Could you check a few things on this model? Use its own coordinates, in mm. Face numbers are marked on the shaded views. A direction names the side the tool comes from. Give positions to 0.01 mm unless a question says otherwise; leave off trailing zeros. Write each loop counter-clockwise with the first axis right and the second up, starting at its lowest first coordinate (ties: lowest second). Pieces come first, ordered by that corner, then holes. Notation, with made-up numbers: (-17, 29) -> (18, 29) arc R18 ccw to (18, 43) -> close; hole circle Ø10 at (62.25, 74.5). An arc over 180 degrees is marked (long way). Write item = value, one per line. Start each with the question number.
```python
from build123d import *

# Parameters (mm, degrees)
F0_W     = 96
F0_H     = 50
F1_DEPTH = 6
F2_R     = 5
F3_W     = 76
F3_H     = 45
F4_DEPTH = 2
F6_DEPTH = 25


with BuildPart() as f1:
    # F0 (on Top) → F1 (new body)
    with BuildSketch(Plane.XY):
        with Locations((48, 25)):
            Rectangle(F0_W, F0_H)
    extrude(amount=F1_DEPTH)

    # F2
    f2_edges = [f1.edges().sort_by_distance(p)[0] for p in [
        (96, 50, 3),
        (96, 0, 3),
        (0, 50, 3),
        (0, 0, 3),
    ]]
    fillet(f2_edges, radius=F2_R)

    # F3 (on Top) → F4 (cut)
    with BuildSketch(Plane.XY):
        with Locations((48, 27.5)):
            Rectangle(F3_W, F3_H)
    extrude(amount=F4_DEPTH, mode=Mode.SUBTRACT)

    # F5 (on face) → F6 (cut)
    with BuildSketch(Plane.XY.offset(6)):
        with BuildLine():
            Line((81, 42), (15, 42))
            ThreePointArc((15, 42), (13.585786, 41.414214), (13, 40))
            Line((13, 40), (13, 10))
            ThreePointArc((13, 10), (13.585786, 8.585786), (15, 8))
            Line((15, 8), (81, 8))
            ThreePointArc((81, 8), (82.414214, 8.585786), (83, 10))
            Line((83, 10), (83, 40))
            ThreePointArc((83, 40), (82.414214, 41.414214), (81, 42))
        make_face()
    extrude(amount=-F6_DEPTH, mode=Mode.SUBTRACT)


solid = f1.part
```
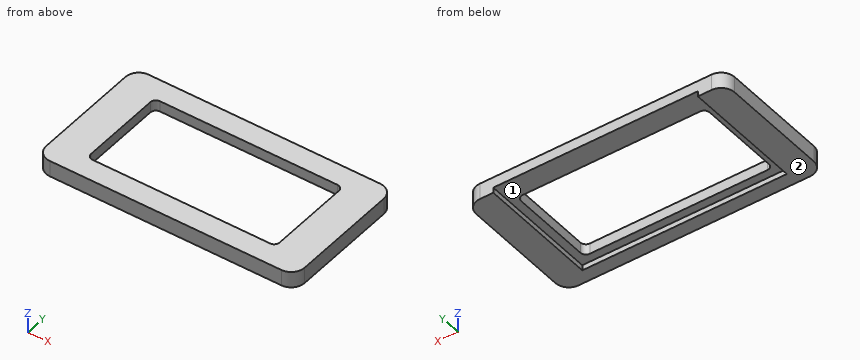
(1) I'm going to push a flat-ended pin straight in: pin 1 (1 mm diameter, centred on x = 59, z = 0.5, fed in from +Y). Where does the tip first touch, or does it pass through?
(2) On a 3-axis mill with a long thin cutter (end or side, diameter ignored), from which of +Z, -Z, +X, -X, +Y, -Y can I reach the whole of each face in a straight line? I mean the marked faces 1 and 2. Say none if no direction works.
(3) Imagine slicing it at C-C (z = 5.1). Please give me the cut outline in (x, y).
(4) Imagine slicing it at A-A (x = 69). Please give me the cut outline in (y, z), then the cut area to 3 significant figures.
(5) If I drill on line 1 along Y through (x, z) = (47.5, 4.65); line 2 along X through (y, z) = (16.5, 4.75); line 3 along X through (y, z) = (43.5, 0.95), over which ranges is the centre line in solid material (lowest first)? Write a range as from..to.
(6) Imagine slicing it at B-B (y = 14). Please give me the cut outline in (x, z), then the cut area to 3 significant figures.
Answers below:
q1.pin_1 = 5
q2.face_1 = -Z, +Y
q2.face_2 = -Z, +X, -X, +Y, -Y
q3.outline = (0, 5) arc R5 ccw to (5, 0) -> (91, 0) arc R5 ccw to (96, 5) -> (96, 45) arc R5 ccw to (91, 50) -> (5, 50) arc R5 ccw to (0, 45) -> close; hole (13, 10) arc R2 ccw to (15, 8) -> (81, 8) arc R2 ccw to (83, 10) -> (83, 40) arc R2 ccw to (81, 42) -> (15, 42) arc R2 ccw to (13, 40) -> close
q4.outline = (0, 0) -> (5, 0) -> (5, 2) -> (8, 2) -> (8, 6) -> (0, 6) -> close; (42, 2) -> (50, 2) -> (50, 6) -> (42, 6) -> close
q4.area = 74.0 mm^2
q5.line_1 = 0..8, 42..50
q5.line_2 = 0..13, 83..96
q5.line_3 = 0..10, 86..96
q6.outline = (0, 0) -> (10, 0) -> (10, 2) -> (13, 2) -> (13, 6) -> (0, 6) -> close; (83, 2) -> (86, 2) -> (86, 0) -> (96, 0) -> (96, 6) -> (83, 6) -> close
q6.area = 144 mm^2
